Could you check a few things on this model? Use its own coordinates, in mm. Face numbers are marked on the shaded views. A direction names the side the tool comes from. Round coordinates to 2 decimals unless told otherwise and drop trailing zeros. Order: outer loops, then holes, each group sorted by start corner. A loop starts at its lowest first (then second) coordinate and runs counter-clockwise, first axis right, second up. Notation, with made-up numbers: (61.5, 12) - (84.5, 12) arc R25 cw to (84.5, 40) - close; hole circle Ø6 at (17.25, 26). An arc over 180 degrees is marked (long way). Use one line per item in the form item = value.
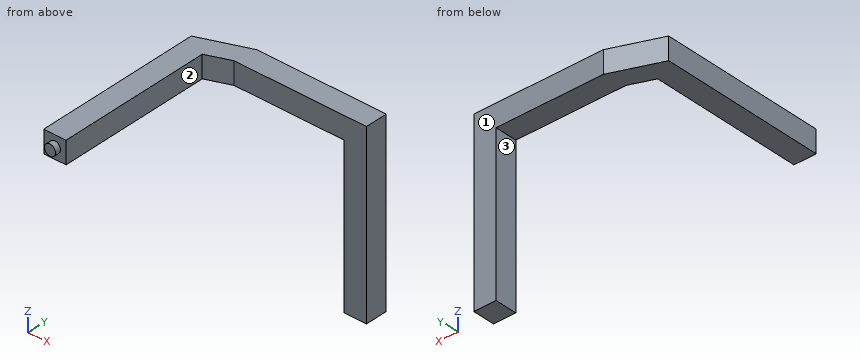
from build123d import *

# Parameters (mm, degrees)
SKETCH1_W           = 100
SKETCH1_H           = 100
BOSS_EXTRUDE1_DEPTH = 800
SKETCH2_W           = 100
SKETCH2_H           = 100
BOSS_EXTRUDE2_DEPTH = 700
CUT_EXTRUDE1_DEPTH  = 801
BOSS_EXTRUDE3_DEPTH = 100
SKETCH5_R           = 25
BOSS_EXTRUDE4_DEPTH = 25


with BuildPart() as part:
    # Sketch1 → Boss-Extrude1 (new body)
    with BuildSketch(Plane.XY):
        with Locations((50, 50)):
            Rectangle(SKETCH1_W, SKETCH1_H)
    extrude(amount=BOSS_EXTRUDE1_DEPTH)

    # Sketch2 → Boss-Extrude2 (add)
    with BuildSketch(Plane(origin=(0, 0, 0), x_dir=(0, 0, -1), z_dir=(1, 0, 0))):
        with Locations((-750, 50)):
            Rectangle(SKETCH2_W, SKETCH2_H)
    extrude(amount=-BOSS_EXTRUDE2_DEPTH)

    # Sketch3 → Cut-Extrude1 (cut, through all)
    with BuildSketch(Plane.XY):
        Polygon((-481.374152596, 100), (-700, 15.631226575), (-700, 100), align=None)
    extrude(amount=CUT_EXTRUDE1_DEPTH, mode=Mode.SUBTRACT)

    # Sketch4 → Boss-Extrude3 (add)
    with BuildSketch(Plane.XY.offset(800)):
        Polygon((-493.990986432, 0), (-600, -41.564522078), (-600, -730.356100977), (-700, -730.356100977), (-700, 0), align=None)
    extrude(amount=-BOSS_EXTRUDE3_DEPTH)

    # Sketch5 → Boss-Extrude4 (add)
    with BuildSketch(Plane(origin=(0, -730.356100977, 0), x_dir=(-1, 0, 0), z_dir=(0, -1, 0))):
        with Locations((650, -750)):
            Circle(SKETCH5_R)
    extrude(amount=BOSS_EXTRUDE4_DEPTH)


solid = part.part
Item 1: Imagine slicing it at A-A on z = 750. Please give me the cut outline in (x, y), plus the area to 3 significant figures.
Found:
outline = (-700, -730.36) - (-675, -730.36) - (-675, -755.36) - (-625, -755.36) - (-625, -730.36) - (-600, -730.36) - (-600, -41.56) - (-493.99, 0) - (100, 0) - (100, 100) - (-481.37, 100) - (-700, 15.63) - close
area = 147,000 mm2
Item 2: Imagine slicing it at C-C on x = -650. Please give me the cut outline in (y, z), plus the area to 3 significant figures.
Found:
outline = (-755.36, 725) - (-730.36, 725) - (-730.36, 700) - (34.93, 700) - (34.93, 800) - (-730.36, 800) - (-730.36, 775) - (-755.36, 775) - close
area = 77,800 mm2
Item 3: Imagine slicing it at D-D on x = -45. Please give me the cut outline in (y, z).
Found:
outline = (0, 700) - (100, 700) - (100, 800) - (0, 800) - close
Item 4: Imagine slicing it at B-B on y = -311.5. Please give me the cut outline in (x, z), plus the area to 3 significant figures.
Found:
outline = (-700, 700) - (-600, 700) - (-600, 800) - (-700, 800) - close
area = 10,000 mm2
Item 5: Will this pin go through, and if not, where does the flat tip stop? P1, Ø6, axis at x = -47.5, y = 7, coming from the -Z side.
Found:
P1 = 700
Item 6: For the marked faces 1, 2 and 3, which set-ups out of +Z, -Z, +X, -X, +Y, -Y let a thin tool reach every point of the face, with its end or its side?
Found:
face_1 = +Z, -Z, +X, -X, +Y
face_2 = +Z, -Z, +X, -Y
face_3 = -Z, -X, +Y, -Y
Item 7: I need wall thicknesses on L1, parallel to Z at x = -609.5, y = 2.5; L2, parallel to X at y = -193, z = 738; L3, parallel to Y at x = 68, z = 478.5. Which ranges of each line are inside material? Lowest first, please.
Found:
L1 = 700 to 800
L2 = -700 to -600
L3 = 0 to 100
